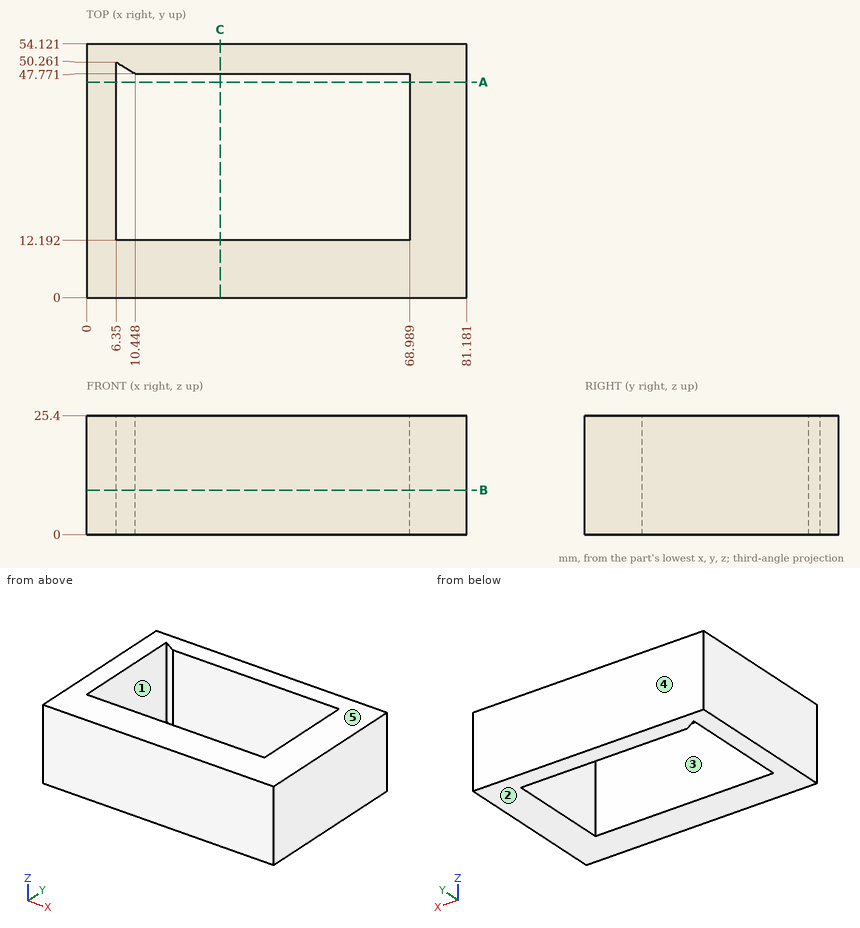
Check sheet for the drawn part. Datum: minimum x, y, z corner. Units: mm. A direction names the side the tool comes from. Give positions to 0.01 mm unless a question says otherwise; leave off trailing zeros. Write each loop counter-clockwise with the first axis right and the second up, starting at its lowest first coordinate (ties: lowest second). Pieces come first, ordered by that corner, then holes. Notation, with made-up numbers: (51, 16.5) -> (105, 16.5) arc R20 cw to (105, 32.5) -> close; hole circle Ø1 at (-38, 8). An arc over 180 degrees is marked (long way). Use one line per item in the form item = value. Start each with the question number.
1. Section check B-B (z = 9.5). Record the cut outline in (x, y).
2. Mould release check, pull along Y, two halves, no side actions. Record for the marked faces 3, 4 and 5: pulls with the +Y half, pulls with the -Y half, needs draft (parallel to the pull), parting line crosses it, or undercut.
3. Section check A-A (y = 46). Record the cut outline in (x, z), and give its area (3 significant figures).
4. Access from +Z, -Z, +X, -X, +Y, -Y to the whole of each face (thin tool, end or side, straight path). Record for the marked faces 1 and 2.
5. Section check C-C (x = 28.5). Record the cut outline in (y, z), and give its area (3 significant figures).
6. Thickness scan on line 1 along Y through (x, z) = (59.5, 21.5); line 2 along X through (y, z) = (32.5, 1.75); line 3 along Y through (x, z) = (10, 20.5). Record the ranges inside material, lowest first. Write a range as from..to.
Conclusion:
q1.outline = (0, 0) -> (81.18, 0) -> (81.18, 54.12) -> (0, 54.12) -> close; hole (6.35, 12.19) -> (68.99, 12.19) -> (68.99, 47.77) -> (10.45, 47.77) -> (6.35, 50.26) -> close
q2.face_3 = undercut
q2.face_4 = pulls with the +Y half
q2.face_5 = needs draft
q3.outline = (0, 0) -> (6.35, 0) -> (6.35, 25.4) -> (0, 25.4) -> close; (68.99, 0) -> (81.18, 0) -> (81.18, 25.4) -> (68.99, 25.4) -> close
q3.area = 471 mm²
q4.face_1 = +Z, -Z
q4.face_2 = -Z, +X, -X, +Y, -Y
q5.outline = (0, 0) -> (12.19, 0) -> (12.19, 25.4) -> (0, 25.4) -> close; (47.77, 0) -> (54.12, 0) -> (54.12, 25.4) -> (47.77, 25.4) -> close
q5.area = 471 mm²
q6.line_1 = 0..12.19, 47.77..54.12
q6.line_2 = 0..6.35, 68.99..81.18
q6.line_3 = 0..12.19, 48.04..54.12
